Model file for the job. Use its own axes, mm. A direction names the side the tool comes from. Round coordinates to 2 decimals unless told otherwise and drop trailing zeros. Order: outer loops, then holes, each group sorted by start corner. A loop starts at its lowest first (then second) coordinate and runs counter-clockwise, first axis right, second up. Notation, with made-up numbers: M -20.75,41 L 0.25,41 A19 ccw 0.25,49 Z; hole C -29.5,-19.75 d8. An arc over 180 degrees is marked long. Return JSON: item names as keys, results as strings. Group by question number.
Item 1: Which spindle directions (+Z, -Z, +X, -X, +Y, -Y) get a long thin tool onto all of the face, cutting with end or side? Do faces 1 (the face through (12.7, 0, -4)), 2 (the face through (0, 9.525, -4)). Say none if no direction does.
Item 2: Pin check, flat tip, straight feed: pin 1 Ø6 at (x, y) = (-8, 5) entering from -Z. Stop position of the tip, or through.
Item 3: Pull direction X, two halves, no side cores. Call faces 3 (the face through (0, -9.525, -4)), 4 (the face through (-0.18, -11.11, 298.63)), 5 (the face through (-12.7, 0, -4)): pulls with the +X half, pulls with the -X half, needs draft (parallel to the pull), parting line crosses it, or undercut.
Item 4: Slice it at B-B on y = 1.5. Write the cut outline in (x, z) (3 decimals).
Item 5: Probe line 1 along X through (y, z) = (0.5, -113) (3 decimals); line 2 along Z through (x, y) = (6.75, -11.5). List the from-to ranges inside material, lowest first.
Item 6: Slice it at C-C on z = 122. Write the cut outline in (x, y) (3 decimals).
Item 7: Slice it at A-A on x = 4.75. Write the cut outline in (y, z) (3 decimals), then the cut area to 3 significant figures.
Autodesk Inventor part; units mm, degrees
ref_plane "YZ Plane" through (0, 0, 0) normal (1, 0, 0) x (0, 1, 0)
ref_plane "XZ Plane" through (0, 0, 0) normal (0, 1, 0) x (-1, 0, 0)
ref_plane "XY Plane" through (0, 0, 0) normal (0, 0, 1) x (1, 0, 0)
sketch "Sketch1" plane through (0, 0, 0) normal (0, 0, 1) x (1, 0, 0)
  line L0 (-17.78, 0) -> (17.78, 0)
  line L1 (0, -17.78) -> (0, 17.78)
  line L2 (-12.7, 12.7) -> (12.7, 12.7)
  line L3 (12.7, 12.7) -> (12.7, -12.7)
  line L4 (12.7, -12.7) -> (-12.7, -12.7)
  line L5 (-12.7, -12.7) -> (-12.7, 12.7)
  line L6 (9.525, 9.525) -> (-9.525, 9.525)
  line L7 (-9.525, 9.525) -> (-9.525, -9.525)
  line L8 (-9.525, -9.525) -> (9.525, -9.525)
  line L9 (9.525, -9.525) -> (9.525, 9.525)
  point P0 (0, 0)
  point P1 (-12.7, 0)
  point P2 (0, 12.7)
  dimension "d0" = 25.4
  dimension "d1" = 3.175
extrude "Extrusion1" add sketch "Sketch1" along normal mid plane 622.3 contours L5 L2 L1 L6 L7 L0 | L0 L7 L8 L1 L4 L5 | L1 L8 L9 L0 L3 L4 | L2 L3 L0 L9 L6 L1
sketch "Sketch3" plane through (-12.7, 12.7, 311.15) normal (0, 1, 0) x (1, 0, 0)
  line L0 (0, 0) -> (25.4, 0)
  line L1 (25.4, 0) -> (25.4, 622.3)
  line L2 (0, 622.3) -> (0, 0)
  line L3 (0, 311.15) -> (25.4, 311.15) construction
  line L4 (0, 0) -> (25.4, 25.4)
  line L5 (25.4, 0) -> (25.4, 25.4)
  line L6 (0, 0) -> (25.4, 0)
  line L7 (0, 622.3) -> (25.4, 596.9)
  line L8 (25.4, 622.3) -> (25.4, 596.9)
  line L9 (0, 622.3) -> (25.4, 622.3)
  point P0 (12.7, 311.15)
  dimension "d7" = 45
extrude "Extrusion3" cut sketch "Sketch3" against normal through all contours L4 L1 L0 | L9 L1 L7
properties part number "tubing_template_0.125" material "Aluminum-6061"
Output values:
{
 "1": {"face 1": "+Z, -Z, +X, +Y, -Y", "face 2": "+Z, -Z"},
 "2": {"pin 1": "z = -309.45"},
 "3": {"face 3": "undercut", "face 4": "pulls with the +X half", "face 5": "pulls with the -X half"},
 "4": {"outline": "M -12.7,-311.15 L -9.525,-307.975 L -9.525,307.975 L -12.7,311.15 Z; M 9.525,-288.925 L 12.7,-285.75 L 12.7,285.75 L 9.525,288.925 Z"},
 "5": {"line 1": "-12.7 to -9.525, 9.525 to 12.7", "line 2": "-291.7 to 291.7"},
 "6": {"outline": "M -12.7,-12.7 L 12.7,-12.7 L 12.7,12.7 L -12.7,12.7 Z; hole M -9.525,-9.525 L 9.525,-9.525 L 9.525,9.525 L -9.525,9.525 Z"},
 "7": {"outline": "M -12.7,-293.7 L -9.525,-293.7 L -9.525,293.7 L -12.7,293.7 Z; M 9.525,-293.7 L 12.7,-293.7 L 12.7,293.7 L 9.525,293.7 Z", "area": "3,730 mm²"}
}
